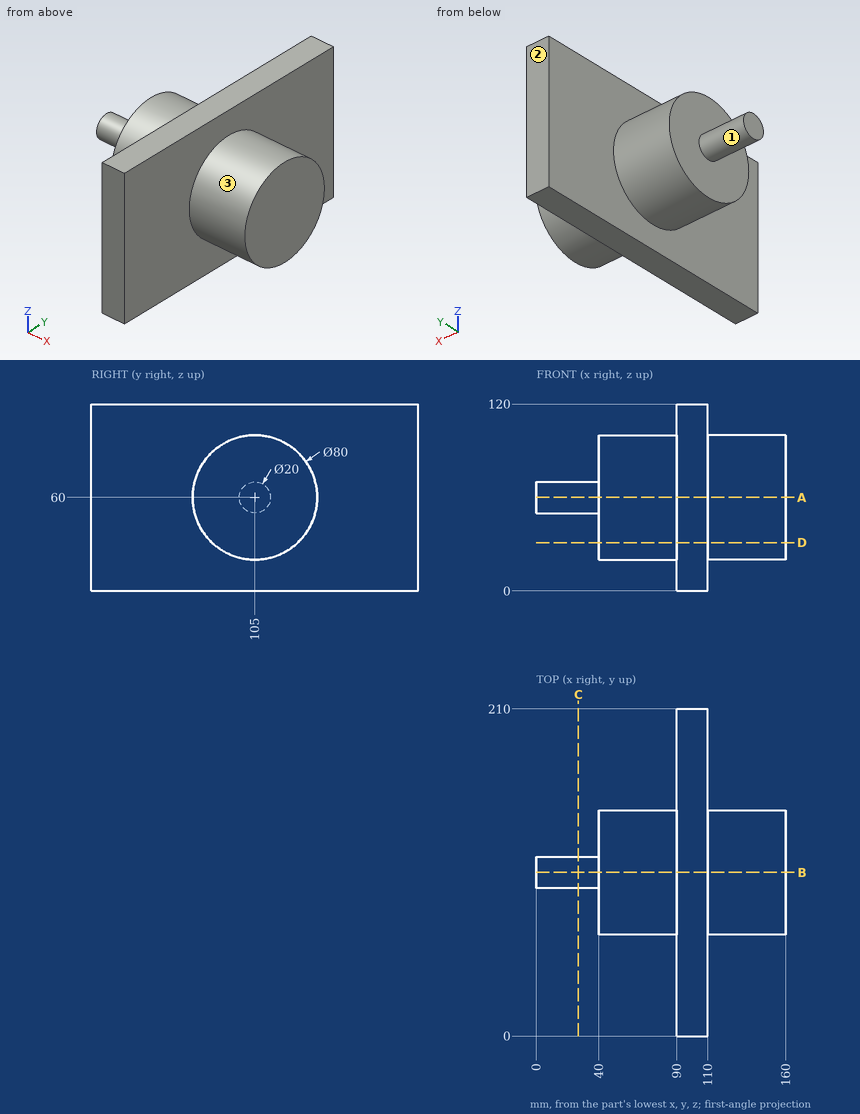
Could you check a few things on this drawing? It's one solid part, dimensions in mm from its lowest x, y, z. A direction names the side the tool comes from. Give positions to 0.01 mm unless a question says otherwise; leave off trailing zeros. Write each loop counter-clockwise with the first axis right and the second up, starting at its lowest first coordinate (ties: lowest second). Pieces come first, ordered by that corner, then holes.
(1) Will these pins go through, and if not, where does the flat tip stop? pin 1 (5 mm diameter, centred on x = 52, z = 62, fed in from +Y); pin 2 (12 mm diameter, centred on y = 50, z = 16.5, fed in from +X); pin 3 (5 mm diameter, centred on x = 118, z = 33.5, fed in from +Y).
Output values:
pin 1: stops at y = 145
pin 2: stops at x = 110
pin 3: stops at y = 137
(2) On a 3-axis mill with a long thin cutter (end or side, diameter ignored), from which of +Z, -Z, +X, -X, +Y, -Y can I reach the whole of each face in a straight line? I mean the marked faces 1, 2 and 3. Say none if no direction works.
Output values:
face 1: -X
face 2: +Z, -Z, +X, -X, +Y
face 3: +X
(3) Imagine slicing it at A-A, the plane z = 60. Write out the boundary of the cut face in (x, y), and give its area (3 significant figures).
Output values:
outline: (0, 95) - (40, 95) - (40, 65) - (90, 65) - (90, 0) - (110, 0) - (110, 65) - (160, 65) - (160, 145) - (110, 145) - (110, 210) - (90, 210) - (90, 145) - (40, 145) - (40, 115) - (0, 115) - close
area: 13,000 mm2
(4) If I drill on L1, parallel to X at y = 105, z = 26; L2, parallel to X at y = 139, z = 100; L3, parallel to Y at x = 64.5, z = 58.5, over which ranges is the centre line in solid material (lowest first)?
Output values:
L1: x = 40 to 160
L2: x = 90 to 110
L3: y = 65.03 to 144.97
(5) Imagine slicing it at B-B, the plane y = 105. Write out the boundary of the cut face in (x, z).
Output values:
outline: (0, 50) - (40, 50) - (40, 20) - (90, 20) - (90, 0) - (110, 0) - (110, 20) - (160, 20) - (160, 100) - (110, 100) - (110, 120) - (90, 120) - (90, 100) - (40, 100) - (40, 70) - (0, 70) - close
(6) Imagine slicing it at D-D, the plane z = 31. Write out the boundary of the cut face in (x, y), and give its area (3 significant figures).
Output values:
outline: (40, 77.45) - (90, 77.45) - (90, 0) - (110, 0) - (110, 77.45) - (160, 77.45) - (160, 132.55) - (110, 132.55) - (110, 210) - (90, 210) - (90, 132.55) - (40, 132.55) - close
area: 9,710 mm2
(7) Imagine slicing it at C-C, the plane x = 27. Write out the boundary of the cut face in (y, z), and give its area (3 significant figures).
Output values:
outline: circle Ø20 at (105, 60)
area: 314 mm2
